Here's the drawing with two shaded views (mm, measured from the low corner). I have some questions. A direction names the side the tool comes from. Round coordinates to 2 decimals unless told otherwise and drop trailing zeros. Order: outer loops, then holes, each group sorted by start corner. A loop starts at its lowest first (then second) coordinate and runs counter-clockwise, first axis right, second up. Notation, with made-up numbers: (7.5, -8.5) - (17.5, -8.5) arc R16 cw to (17.5, 5.5) - close; hole circle Ø9 at (49, 65.25). An arc over 180 degrees is marked (long way). One line per item, written item: value.
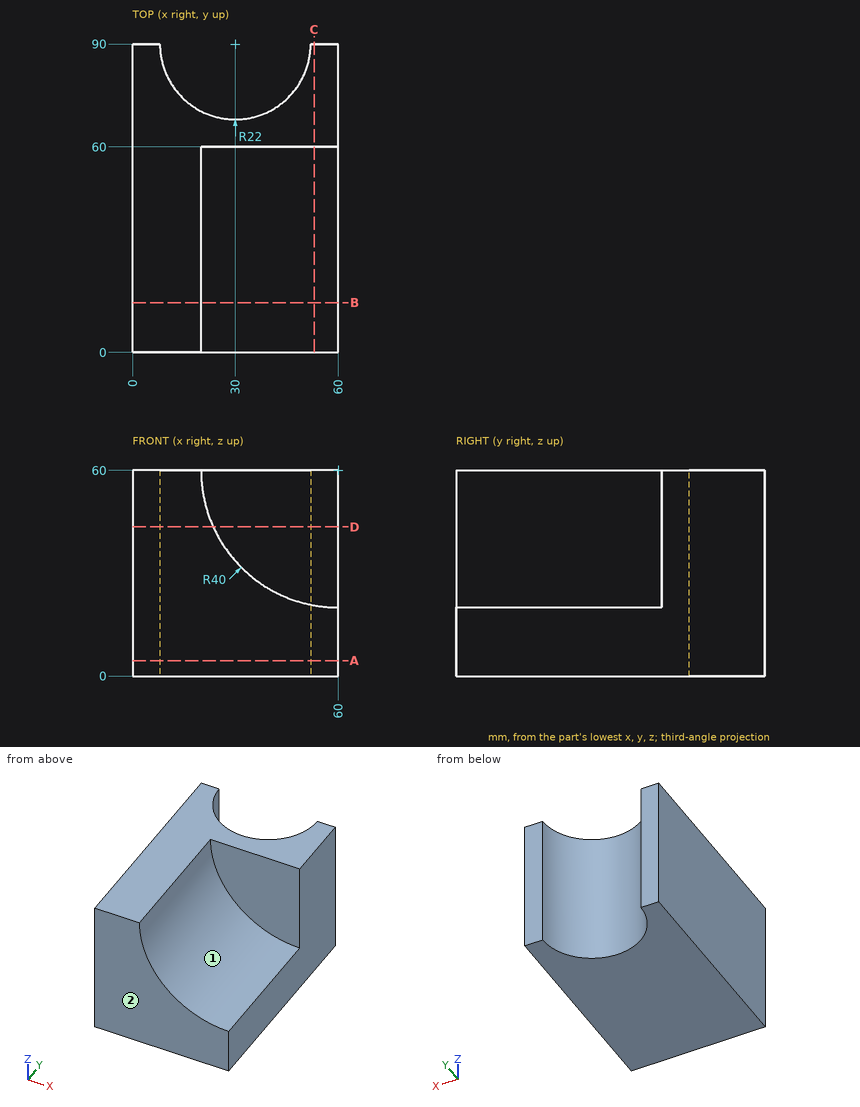
Q1. If we section it at A-A, the plane z = 4.5: Please give me the cut outline in (x, y).
Results list:
outline: (0, 0) - (60, 0) - (60, 90) - (52, 90) arc R22 cw to (8, 90) - (0, 90) - close
Q2. Will these pins go through, and if not, where does the flat tip stop? pin 1 (6 mm diameter, centred on y = 54.5, z = 38, fed in from +X) (3 decimals); pin 2 (1.5 mm diameter, centred on x = 51.5, y = 13.5, fed in from +Z); pin 3 (8 mm diameter, centred on x = 34, z = 18.5, fed in from +Y).
Results list:
pin 1: x = 28.775
pin 2: z = 21.08
pin 3: y = 69.51
Q3. If I drill on line 1 along Y through (x, z) = (30, 55); line 2 along X through (y, z) = (71, 37.5); line 3 along Y through (x, z) = (54, 56.5), over which ranges is the centre line in solid material (lowest first)?
Results list:
line 1: 60 to 68
line 2: 0 to 18.91, 41.09 to 60
line 3: 60 to 90
Q4. Which directions (+Z, -Z, +X, -X, +Y, -Y) give clear straight access to the entire face, cutting with the end or side of a thin tool? Please do the marked faces 1 and 2.
Results list:
face 1: +Z, +X, -Y
face 2: +Z, -Z, +X, -X, -Y
Q5. If we section it at B-B, the plane y = 14.5: Please give me the cut outline in (x, z), then the cut area to 3 significant figures.
Results list:
outline: (0, 0) - (60, 0) - (60, 20) arc R40 cw to (20, 60) - (0, 60) - close
area: 2,340 mm²
Q6. If we section it at D-D, the plane z = 43.5: Please give me the cut outline in (x, y), then the cut area to 3 significant figures.
Results list:
outline: (0, 0) - (23.56, 0) - (23.56, 60) - (60, 60) - (60, 90) - (52, 90) arc R22 cw to (8, 90) - (0, 90) - close
area: 2,450 mm²
Q7. If we section it at C-C, the plane x = 53: Please give me the cut outline in (y, z), then the cut area to 3 significant figures.
Results list:
outline: (0, 0) - (90, 0) - (90, 60) - (60, 60) - (60, 20.62) - (0, 20.62) - close
area: 3,040 mm²
